Source: CAD feature listing. Evaluate the final solid. Frame: model axes, mm. A direction names the side the tool comes from. Round coordinates to 2 decimals unless told otherwise and drop trailing zeros. Order: outer loops, then holes, each group sorted by start corner. A loop starts at its lowest first (then second) coordinate and runs counter-clockwise, first axis right, second up. Notation, with made-up numbers: (26.5, 9) -> (56.5, 9) arc R27 cw to (56.5, 34) -> close; hole circle Ø5 at (35.25, -28). An arc over 180 degrees is marked (long way). Write item = value, one per line. Start each with the question number.
(1) Cut plane B-B on x = 20.5. Return the cut outline in (y, z).
(2) Cut plane A-A on y = 0. Return the cut outline in (x, z) (3 decimals).
(3) Cut plane C-C on x = 4. Return the cut outline in (y, z), then the cut area to 3 significant figures.
(4) Draft query along X for faces 4 (the face through (-25.616, 0, -4)), 5 (the face through (-17.876, -4.051, 8.993)), 6 (the face through (25.616, 0, -4)), 7 (the face through (6.17, 19.85, 6.46)). Return one class per face: released by +X, released by -X, zero draft, split by the parting line, or undercut.
(5) Contact query for flat-ended pins moving along their axis: pin 1 Ø1 at (x, z) = (7, -0.5) entering from +Y; pin 2 Ø6 at (x, z) = (-2, 0) entering from -Y; pin 3 Ø4 at (x, y) = (-15, -16.5) entering from -Z; pin 4 Ø3 at (x, z) = (12.5, -6.5) entering from +Y. Output: stop coordinate, or through.
(6) Reachability of faces 1 (the face through (-9.916, 11, 7)), 2 (the face through (-6.226, 21.89, -8.732)), 3 (the face through (17.656, -4.051, 8.993)) from +Z, -Z, +X, -X, +Y, -Y: full face, straight path, thin tool, end or side. Return the list, or none.
(7) Ray query, line 1 (Y direction, x = 15, z = -4.5); line 2 (X direction, y = 9.5, z = 10.5); line 3 (X direction, y = 23, z = -8). Return the intervals inside material, ascending.
from build123d import *


with BuildPart() as f1:
    # F0 (on Front) → F1 (revolve)
    with BuildSketch(Plane.XZ):
        with BuildLine():
            Line((-25.6159, 9.616317), (-25.6159, -3.871083))
            Line((-25.6159, -3.871083), (25.6159, -3.871083))
            Line((25.6159, -3.871083), (25.6159, 9.616317))
            Line((25.6159, 9.616317), (9.916342, 9.616317))
            Line((9.916342, 9.616317), (9.916342, 21.528917))
            Line((9.916342, 21.528917), (5.979342, 18.353917))
            ThreePointArc((5.979342, 18.353917), (0, 16.243301), (-5.979342, 18.353917))
            Line((-5.979342, 18.353917), (-9.916342, 21.528917))
            Line((-9.916342, 21.528917), (-9.916342, 9.616317))
            Line((-9.916342, 9.616317), (-25.6159, 9.616317))
        make_face()
    revolve(axis=Axis((0, 0, -3.871083), (1, 0, 0)))


solid = f1.part
Evaluation:
q1.outline = circle Ø26.97 at (0, -3.87)
q2.outline = (-25.616, -17.358) -> (-9.916, -17.358) -> (-9.916, -29.271) -> (-5.979, -26.096) arc R9.525 cw to (5.979, -26.096) -> (9.916, -29.271) -> (9.916, -17.358) -> (25.616, -17.358) -> (25.616, 9.616) -> (9.916, 9.616) -> (9.916, 21.529) -> (5.979, 18.354) arc R9.525 cw to (-5.979, 18.354) -> (-9.916, 21.529) -> (-9.916, 9.616) -> (-25.616, 9.616) -> close
q3.outline = circle Ø41.99 at (0, -3.87)
q3.area = 1,380 mm^2
q4.face_4 = released by -X
q4.face_5 = zero draft
q4.face_6 = released by +X
q4.face_7 = undercut
q5.pin_1 = 23.21
q5.pin_2 = -21.25
q5.pin_3 = through
q5.pin_4 = 13.44
q6.face_1 = -X
q6.face_2 = none
q6.face_3 = +X
q7.line_1 = -13.47 to 13.47
q7.line_2 = -9.92 to 9.92
q7.line_3 = -9.92 to -7.4, 7.4 to 9.92
